Here's the drawing with two shaded views (mm, measured from the low corner). I have some questions. Give positions to 0.01 mm unless a question says otherwise; leave off trailing zeros. Loops run counter-clockwise (first coordinate to the right, second up) from the corner with the lowest first, then second, coordinate; pieces in that order, holes last. Notation, with made-up numbers: (61, 87) -> (88, 87) arc R5 cw to (88, 94) -> close; hole circle Ø7 at (-23, 80). An arc over 180 degrees is marked (long way). Answer in a Markdown table with one row per item. Add a question column.
Item 1: If we section it at B-B (x = 17): Write out the boundary of the cut face in (y, z) (1 decimal).
Item 2: If we section it at D-D (y = 2.5): Write out the boundary of the cut face in (x, z).
Item 3: If I drill on line 1 (X direction, y = 16.02, z = 1.65); line 2 (Y direction, x = 16.02, z = 1.75); line 3 (X direction, y = 14, z = 3.75) (1 decimal), over which ranges is the centre line in solid material (lowest first)?
Item 4: If we section it at C-C (z = 1.6): Write out the boundary of the cut face in (x, y) (1 decimal).
Item 5: For P1, Ø1.5, axis at x = 27, z = 2, coming from the -Y side; P2, Ø1, axis at y = 19, z = 3.5, coming from the -X side, each with a flat end and sliding along its axis, tell me the tip position at first contact or that it passes through.
Item 6: If we section it at A-A (y = 29.5): Write out the boundary of the cut face in (x, z).
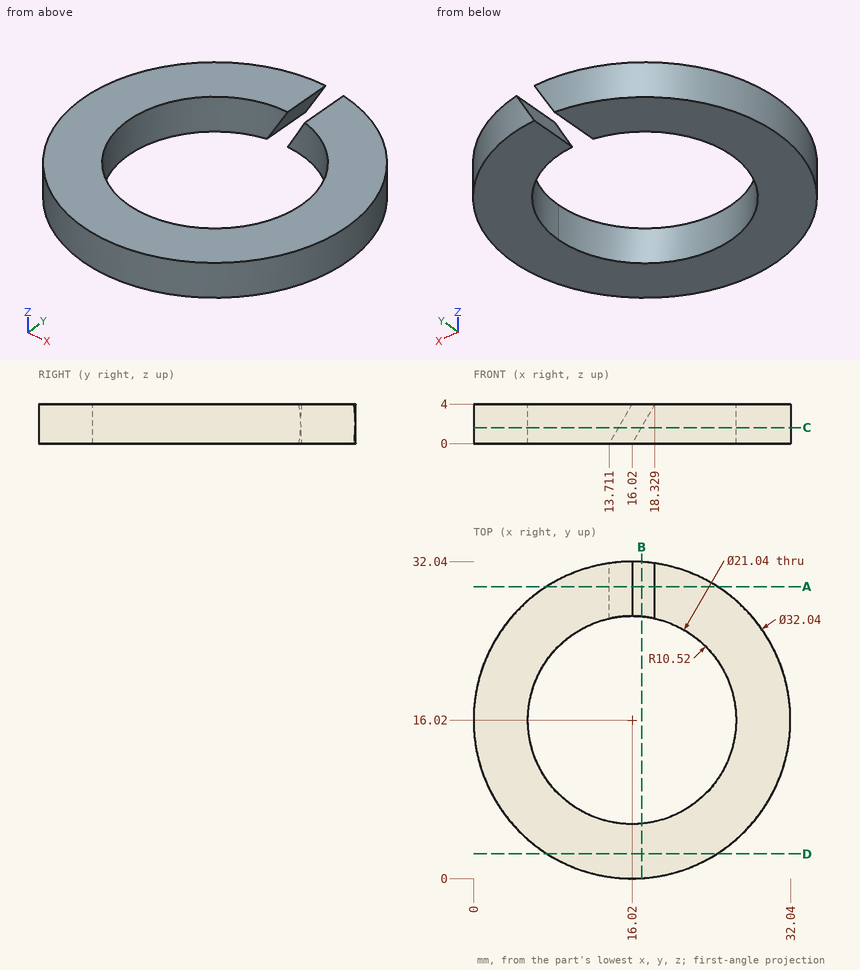
Recorded:
| question | item | result |
|---|---|---|
| 1 | outline | (0, 0) -> (5.5, 0) -> (5.5, 4) -> (0, 4) -> close; (26.5, 0) -> (32, 0) -> (32, 1.7) -> (26.5, 1.7) -> close |
| 2 | outline | (7.43, 0) -> (24.61, 0) -> (24.61, 4) -> (7.43, 4) -> close |
| 3 | line 1 | x = 0 to 5.5, 26.54 to 32.04 |
| 3 | line 2 | y = 0 to 5.5 |
| 3 | line 3 | x = 0.1 to 5.7, 26.3 to 31.9 |
| 4 | outline | (14.6, 26.4) -> (14.6, 32) arc R16 ccw (long way) to (16.9, 32) -> (16.9, 26.5) arc R10.5 cw (long way) to start |
| 5 | P1 | stops at y = 3.69 |
| 5 | P2 | stops at x = 0.19 |
| 6 | outline | (7.36, 0) -> (13.71, 0) -> (16.02, 4) -> (7.36, 4) -> close; (16.02, 0) -> (24.68, 0) -> (24.68, 4) -> (18.33, 4) -> close |
